The model under review builds one solid part; all positions refer to its coordinate system, in mm. A direction names the side the tool comes from. Round coordinates to 2 decimals unless told otherwise and drop trailing zeros. Order: outer loops, then holes, each group sorted by start corner. A loop starts at its lowest first (then second) coordinate and runs counter-clockwise, first axis right, second up. Notation, with made-up numbers: M 57,18 L 73,18 A25 cw 73,35 Z; hole C -24,-13 d2. An arc over 180 degrees is marked long. One line per item, written item: value. Start each with the question number.
from build123d import *

# Parameters (mm, degrees)
EXTRUDE_1_DEPTH          = 15
CUT_EXTRUDE_2_DEPTH      = 2
SKETCH_2_R               = 45
CUT_EXTRUDE_3_DEPTH      = 279.25348156
CUT_EXTRUDE_4_DEPTH      = 279.25348156
CUT_EXTRUDE_4_DEPTH_BACK = 279.25348156
HOLE_WIZARD_M5_1_D       = 4.2
HOLE_WIZARD_M6_1_D       = 5


with BuildPart() as part:
    # 草图1 → 凸台-拉伸1 (new body)
    with BuildSketch(Plane.XY):
        with BuildLine():
            Line((140, 183), (140, 240))
            Line((140, 240), (-140, 240))
            Line((-140, 240), (-140, -240))
            Line((-140, -240), (140, -240))
            Line((140, -240), (140, -183))
            Line((140, -183), (80, -183))
            ThreePointArc((80, -183), (-103, 0), (80, 183))
            Line((80, 183), (140, 183))
        make_face()
        with BuildLine():
            Line((140, -168), (140, 168))
            Line((140, 168), (80, 168))
            ThreePointArc((80, 168), (-88, 0), (80, -168))
            Line((80, -168), (140, -168))
        make_face()
        with BuildLine():
            Line((140, 168), (140, 183))
            Line((140, 183), (80, 183))
            ThreePointArc((80, 183), (-103, 0), (80, -183))
            Line((80, -183), (140, -183))
            Line((140, -183), (140, -168))
            Line((140, -168), (80, -168))
            ThreePointArc((80, -168), (-88, 0), (80, 168))
            Line((80, 168), (140, 168))
        make_face()
    extrude(amount=EXTRUDE_1_DEPTH)

    # 草图1<4> → 切除-拉伸2 (cut)
    with BuildSketch(Plane.XY):
        with BuildLine():
            Line((140, 168), (140, 183))
            Line((140, 183), (80, 183))
            ThreePointArc((80, 183), (-103, 0), (80, -183))
            Line((80, -183), (140, -183))
            Line((140, -183), (140, -168))
            Line((140, -168), (80, -168))
            ThreePointArc((80, -168), (-88, 0), (80, 168))
            Line((80, 168), (140, 168))
        make_face()
    extrude(amount=CUT_EXTRUDE_2_DEPTH, mode=Mode.SUBTRACT)

    # 草图2 → 切除-拉伸3 (cut, through all)
    with BuildSketch(Plane(origin=(0, 0, 0), x_dir=(-1, 0, 0), z_dir=(0, 0, -1))):
        with Locations((-80, 0)):
            Circle(SKETCH_2_R)
    extrude(amount=-CUT_EXTRUDE_3_DEPTH, mode=Mode.SUBTRACT)

    # 草图3 → 切除-拉伸4 (cut, two sides: drawn at the far end of the back side and taken through both)
    with BuildSketch(Plane(origin=(0, 0, 0), x_dir=(-1, 0, 0), z_dir=(0, 0, -1)).offset(-CUT_EXTRUDE_4_DEPTH_BACK)):
        Polygon((140, 240), (-77.846096908, 240), (130, 120), (130, -120), (-77.846096908, -240), (140, -240), align=None)
    extrude(amount=CUT_EXTRUDE_4_DEPTH + CUT_EXTRUDE_4_DEPTH_BACK, mode=Mode.SUBTRACT)

    # M5 螺纹孔1 (through all)
    with Locations(Plane(origin=(0, 0, 0), x_dir=(-1, 0, 0), z_dir=(0, 0, -1))):
        with Locations((-122.426406871, 42.426406871), (-37.573593129, 42.426406871), (-37.573593129, -42.426406871), (-122.426406871, -42.426406871)):
            Hole(HOLE_WIZARD_M5_1_D / 2)

    # M6 螺纹孔1 (through all)
    with Locations(Plane(origin=(130, 175.5, 2), x_dir=(-1, 0, 0), z_dir=(0, 0, -1))):
        with Locations((0, 0), (95.422742415, -5.980017486), (174.097240098, -51.402759902), (219.519982514, -130.077257585), (219.519982514, -220.922742415), (174.097240098, -299.597240098), (95.422742415, -345.019982514), (0, -351)):
            Hole(HOLE_WIZARD_M6_1_D / 2)


solid = part.part
Item 1: Consider section C-C, the plane z = 8.5. Count the separate pieces of the cut face and the enclosed holes in it, then the cut area to 3 significant figures.
Item 2: Consider section B-B, the plane y = 10.5. Give the boundary of the cut face in (x, z).
Item 3: Clearance check with flat-ended pins moving along their axes: P1, Ø6, axis at x = 41.5, z = 12, coming from the -Y side; P2, Ø3, axis at x = -44.1, y = 124.1, coming from the +Z side; P3, Ø6, axis at x = -89.52, y = -45.42, coming from the -Z side. State where each tip first meets the part, or that it passes through.
Item 4: The part is to be moulded in two halves that separate along X. For faces 3 (the cylindrical face through (59.235, -39.923, 7.395)), 4 (the flat face through (140, -3, 7)), 5 (the flat face through (-24.62, 180.84, 7.6)), say which applies: pulls with the +X half, pulls with the -X half, needs draft (parallel to the pull), parting line crosses it, or undercut.
Item 5: Consider section A-A, the plane x = 56. Give the boundary of the cut face in (y, z), then the cut area to 3 significant figures.
Item 6: Machinability: for faces 1 (the flat face through (-90, 1, 2)), 2 (the flat face through (109, 240, 7)), which of the approach directions +Z, -Z, +X, -X, +Y, -Y give a long, thin tool a straight path to every point of the face, cutting with its end or side? Answer none if there is none.
Item 7: Wall thickness on L1, parallel to Y at x = 130, z = 8; L2, parallel to Y at x = -45.5, z = 9.25; L3, parallel to Y at x = 41, z = 12.5: over which ranges is each line inside the solid? List them lowest first.
Item 8: Consider section D-D, the plane x = 7. Give the boundary of the cut face in (y, z).
Computed:
1. separate pieces: 1
1. enclosed holes: 13
1. area: 98,100 mm^2
2. outline: M -130,0 L -102.7,0 L -102.7,2 L -87.67,2 L -87.67,0 L 36.24,0 L 36.24,15 L -130,15 Z; M 123.76,0 L 140,0 L 140,15 L 123.76,15 Z
3. P1: stops at y = -220.75
3. P2: passes through
3. P3: stops at z = 2
4. face 3: undercut
4. face 4: pulls with the +X half
4. face 5: pulls with the -X half
5. outline: M -227.39,0 L -181.42,0 L -181.42,2 L -166.28,2 L -166.28,0 L -38.07,0 L -38.07,15 L -227.39,15 Z; M 38.07,0 L 166.28,0 L 166.28,2 L 181.42,2 L 181.42,0 L 227.39,0 L 227.39,15 L 38.07,15 Z
5. area: 5,620 mm^2
6. face 1: -Z
6. face 2: +Z, -Z, +X, -X, +Y
7. L1: y = -240 to -178, -173 to 173, 178 to 240
7. L2: y = -168.79 to -126.17, -122.03 to 122.03, 126.17 to 168.79
7. L3: y = -218.73 to -22.45, 22.45 to 218.73
8. outline: M -199.1,0 L -167.81,0 L -167.81,2 L -151.31,2 L -151.31,0 L 151.31,0 L 151.31,2 L 167.81,2 L 167.81,0 L 199.1,0 L 199.1,15 L -199.1,15 Z
